Study the drawing (mm; zero at the part's minimum x, y, z) and answer. A direction names the side the tool comes from. Give positions to 0.01 mm unless a question says otherwise; leave off trailing zeros. Order: outer loops, then holes, each group sorted by start corner. A loop starts at its lowest first (then second) coordinate and runs counter-clockwise, first axis right, second up.
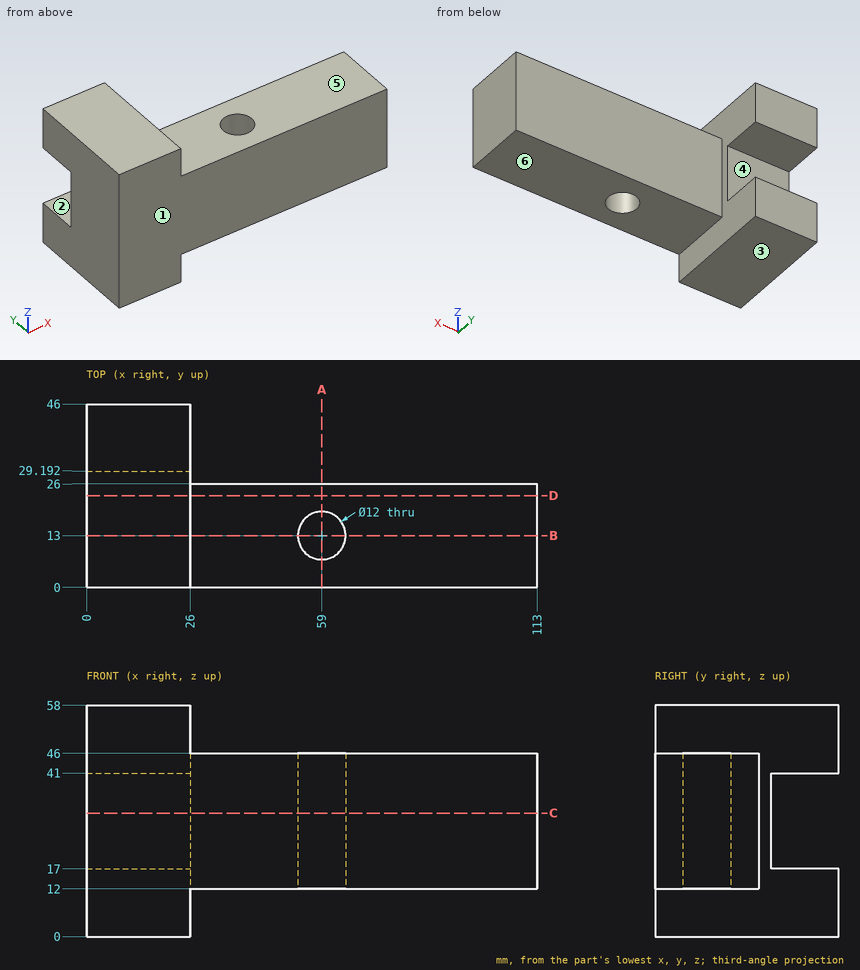
1) A tool of negligible diameter and unlimited length cuts with its end or side. For the marked faces 4, 5 and 6, from which of +Z, -Z, +X, -X, +Y, -Y can it reach the whole face along a straight path? Write none if from no direction.
Geometry says:
face 4: +X, -X, +Y
face 5: +Z, +X, +Y, -Y
face 6: -Z, +X, +Y, -Y
2) Straight lines are drawn through the part: probe 1 along Y at (x, z) = (59, 28.5); probe 2 along Z at (x, y) = (97.5, 8.5); probe 3 along X at (y, z) = (37.5, 6.5). For each, find the intervals that lie inside material, in ascending order.
Geometry says:
probe 1: y = 0 to 7, 19 to 26
probe 2: z = 12 to 46
probe 3: x = 0 to 26
3) Find section B-B (y = 13). Write down the section's boundary in (x, z), then the cut area to 3 significant figures.
Geometry says:
outline: (0, 0) - (26, 0) - (26, 12) - (53, 12) - (53, 46) - (26, 46) - (26, 58) - (0, 58) - close; (65, 12) - (113, 12) - (113, 46) - (65, 46) - close
area: 4,060 mm2
4) Find section C-C (z = 31). Write down the section's boundary in (x, y), then the cut area to 3 significant figures.
Geometry says:
outline: (0, 0) - (113, 0) - (113, 26) - (26, 26) - (26, 29.19) - (0, 29.19) - close; hole circle Ø12 at (59, 13)
area: 2,910 mm2
5) Given P1, Ø15.5, axis at x = 59, y = 13, coming from the +Z side; P2, Ø8, axis at y = 10.5, z = 7, coming from the -X side; P3, Ø10, axis at x = 18, z = 32, coming from the +Y side; P4, Ø13, axis at x = 77.5, y = 10, coming from the -Z side, each flat-ended and moving along its own axis, determine where each tip first touches the part or whether it passes through.
Geometry says:
P1: stops at z = 46
P2: stops at x = 0
P3: stops at y = 29.19
P4: stops at z = 12
6) Find section D-D (y = 23). Write down the section's boundary in (x, z).
Geometry says:
outline: (0, 0) - (26, 0) - (26, 12) - (113, 12) - (113, 46) - (26, 46) - (26, 58) - (0, 58) - close
7) Find section A-A (x = 59). Write down the section's boundary in (y, z), then the cut area to 3 significant figures.
Geometry says:
outline: (0, 12) - (7, 12) - (7, 46) - (0, 46) - close; (19, 12) - (26, 12) - (26, 46) - (19, 46) - close
area: 476 mm2
8) For a pull along Z with two mould halves and no side action, classify the marked faces 1, 2 and 3 as +Z half, -Z half, draft (parallel to the pull), parting line (faces both ways), or undercut.
Geometry says:
face 1: draft
face 2: undercut
face 3: -Z half
